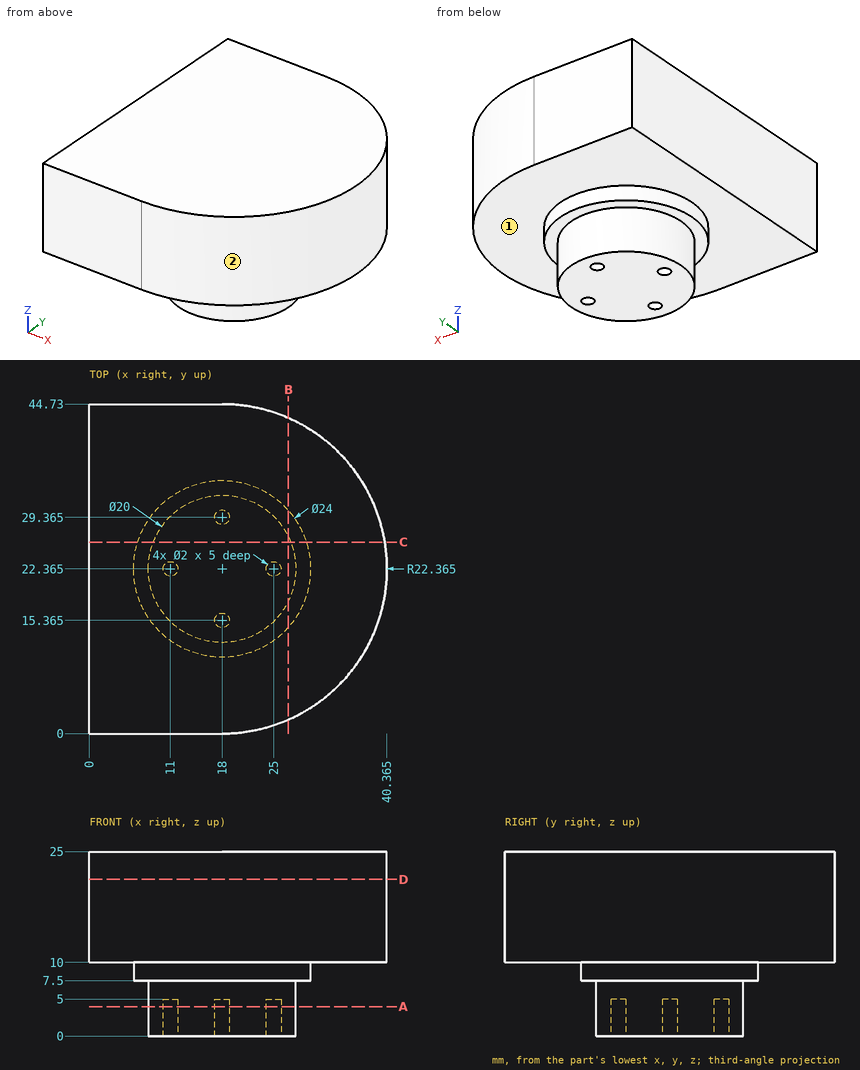
Answer from the drawing. Dimensions are ordinates in mm from the lowest x, y and z of the part. A direction names the side the tool comes from. Round coordinates to 2 decimals unless told otherwise and drop trailing zeros. Loops run counter-clockwise (first coordinate to the right, second up) from the corner with the lowest first, then second, coordinate; pieces in that order, holes last.
(1) The part is cut by section B-B, the plane x = 27. Give the vertices of the cut face in (y, z).
Computed values:
outline: (1.89, 10) - (14.43, 10) - (14.43, 7.5) - (18.01, 7.5) - (18.01, 0) - (26.72, 0) - (26.72, 7.5) - (30.3, 7.5) - (30.3, 10) - (42.84, 10) - (42.84, 25) - (1.89, 25) - close
(2) The part is cut by section C-C, the plane y = 26. Give the vertices of the cut face in (x, z).
Computed values:
outline: (0, 10) - (6.56, 10) - (6.56, 7.5) - (8.68, 7.5) - (8.68, 0) - (27.32, 0) - (27.32, 7.5) - (29.44, 7.5) - (29.44, 10) - (40.07, 10) - (40.07, 25) - (0, 25) - close
(3) Find the intervals of material crossed by L1, parallel to Y at x = 18, z = 1.2 (3 decimals); L2, parallel to Z at x = 19.5, y = 41; L3, parallel to Z at x = 18, y = 12, in increasing order.
Computed values:
L1: y = 12.365 to 14.365, 16.365 to 28.365, 30.365 to 32.365
L2: z = 10 to 25
L3: z = 7.5 to 25
(4) The part is cut by section D-D, the plane z = 21.25. Give the vertices of the cut face in (x, y) (3 decimals), and give its area (3 significant figures).
Computed values:
outline: (0, 0) - (18, 0) arc R22.365 ccw to (18, 44.73) - (0, 44.73) - close
area: 1,590 mm2
(5) Each of these flat-tipped pins is pushed along its axis until it touches: P1, Ø12, axis at x = 9, y = 7.5, coming from the -Z side; P2, Ø2, axis at y = 11, z = 13, coming from the +X side; P3, Ø8, axis at y = 40, z = 9.5, coming from the +X side. Where does it stop, or does it pass through?
Computed values:
P1: stops at z = 7.5
P2: stops at x = 37.82
P3: stops at x = 35.7
(6) For the marked faces 1 and 2, determine the directions among +Z, -Z, +X, -X, +Y, -Y from which every point of the face is accessible in a straight line to the end or side of a thin tool.
Computed values:
face 1: -Z
face 2: +Z, -Z, +X
(7) The part is cut by section A-A, the plane z = 4. Give the vertices of the cut face in (x, y) (3 decimals), and give its area (3 significant figures).
Computed values:
outline: circle Ø20 at (18, 22.365); hole circle Ø2 at (11, 22.365); hole circle Ø2 at (18, 15.365); hole circle Ø2 at (18, 29.365); hole circle Ø2 at (25, 22.365)
area: 302 mm2
